Model file for the job. Use its own axes, mm. Coordinates: 2 decimals unless noted, no trailing zeros. Order: outer loops, then holes, each group sorted by start corner. A loop starts at its lowest first (then second) coordinate and runs counter-clockwise, first axis right, second up. Notation, with made-up numbers: M 68.25,15.5 L 74.25,15.5 A4 ccw 74.25,20.5 Z; hole C 81,-20.5 d4. An arc over 180 degrees is marked long. Return JSON: item names as keys, results as strings.
```python
from build123d import *

# Parameters (mm, degrees)
SKETCH2_R           = 40
BOSS_EXTRUDE2_DEPTH = 10
SKETCH3_R           = 40
BOSS_EXTRUDE4_DEPTH = 155
BOSS_EXTRUDE4_TAPER = 7
FILLET4_R           = 10


with BuildPart() as part:
    # Sketch2 → Boss-Extrude2 (new body)
    with BuildSketch(Plane(origin=(0, 0, 0), x_dir=(1, 0, 0), z_dir=(0, 1, 0))):
        with Locations(Location((0, 0, 0), (0, 0, 270))):
            Circle(SKETCH2_R)
    extrude(amount=BOSS_EXTRUDE2_DEPTH)

    # Sketch3 → Boss-Extrude4 (add)
    with BuildSketch(Plane(origin=(0, 10, 0), x_dir=(1, 0, 0), z_dir=(0, 1, 0))):
        with Locations(Location((0, 0, 0), (0, 0, 270))):
            Circle(SKETCH3_R)
    extrude(amount=BOSS_EXTRUDE4_DEPTH, taper=BOSS_EXTRUDE4_TAPER)

    # Fillet4
    fillet4_edges = [part.edges().sort_by_distance(p)[0] for p in [
        (0, 0, -40),
    ]]
    fillet(fillet4_edges, radius=FILLET4_R - 0.0001)  # a hair under: the kernel refuses the full size


solid = part.part
```
Item 1: Saw through at C-C (y = 128.5). Write the cut outline in (x, z).
Check result:
{"outline": "C 0,0 d50.9"}
Item 2: Wall check: line 1 (X direction, y = 89.5, z = -20.5); line 2 (X direction, y = 121, z = 11); line 3 (Z direction, x = 25, y = 21). Give the ranges that are in metal, low to high.
Check result:
{"line 1": "x = -22.23 to 22.23", "line 2": "x = -23.97 to 23.97", "line 3": "z = -29.47 to 29.47"}
Item 3: Drop flat-ended pins along their axis: pin 1 Ø12 at (x, y) = (-23, 26.5) entering from +Z; pin 2 Ø8 at (y, z) = (19.5, -0.5) entering from +X; pin 3 Ø8 at (x, y) = (23, 23.5) entering from -Z. Give the stop position or say it passes through.
Check result:
{"pin 1": "stops at z = 34.07", "pin 2": "stops at x = 39.32", "pin 3": "stops at z = -33.37"}
Item 4: Saw through at B-B (y = 101.5). Write the cut outline in (x, z), and give its area (3 significant figures).
Check result:
{"outline": "C 0,0 d57.53", "area": "2,600 mm2"}
